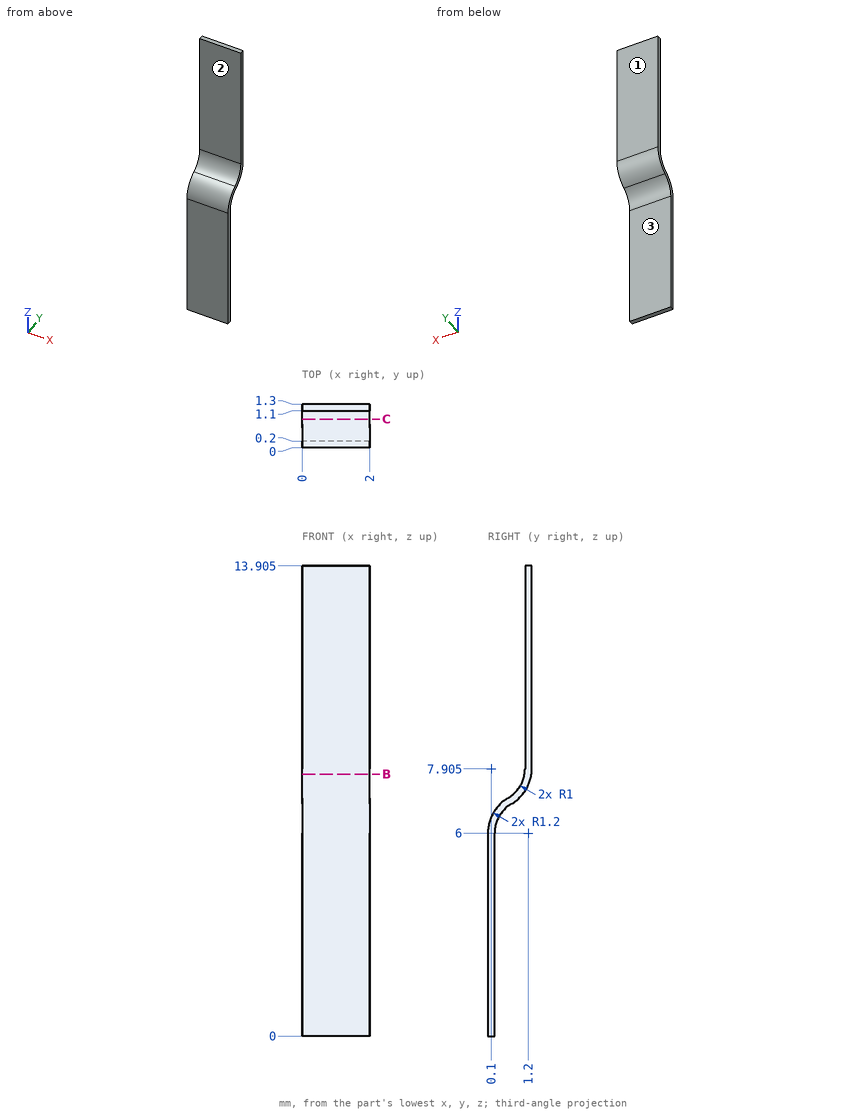
Source: three-view drawing plus pictorial views. Frame: mm from the lowest corner of the part. A direction names the side the tool comes from. Round coordinates to 2 decimals unless told otherwise and drop trailing zeros. Order: outer loops, then holes, each group sorted by start corner. A loop starts at its lowest first (then second) coordinate and runs counter-clockwise, first axis right, second up. Notation, with made-up numbers: M 35,70 L 50,70 A18 ccw 50,83 Z; hole C 79,50 d9. An arc over 180 degrees is marked long. One line per item, written item: value.
(1) Pin query (flat end, axial travel): P1, Ø0.6, axis at x = 1, z = 12, coming from the -Y side. Return the tip coordinate at first contact, or that it passes through.
Result sheet:
P1: y = 1.1
(2) Reachability of the marked faces 1, 2 and 3 from +Z, -Z, +X, -X, +Y, -Y: full face, straight path, thin tool, end or side. Return the list, or none.
Result sheet:
face 1: +Z, -Z, +X, -X, +Y
face 2: +Z, +X, -X, -Y
face 3: -Z, +X, -X, +Y
(3) Cut plane C-C (y = 0.85). Return the cut outline in (x, z).
Result sheet:
outline: M 0,6.97 L 2,6.97 L 2,7.24 L 0,7.24 Z
(4) Line query: probe 1 along Y at (x, z) = (0.25, 1.5); probe 2 along Y at (x, z) = (1.9, 11.5); probe 3 along Z at (x, y) = (1.9, 0.45) (1 decimal). Output: solid intervals per line, ascending. Write a range as [from, to].
Result sheet:
probe 1: [0, 0.2]
probe 2: [1.1, 1.3]
probe 3: [6.7, 6.9]
(5) Cut plane B-B (z = 7.75). Return the cut outline in (x, y).
Result sheet:
outline: M 0,1.09 L 2,1.09 L 2,1.29 L 0,1.29 Z
